```python
from build123d import *

# Parameters (mm, degrees)
BOSS_EXTRUDE1_DEPTH = 90
SKETCH3_R           = 13.36858006
BOSS_EXTRUDE2_DEPTH = 550
SKETCH4_R           = 30
CUT_EXTRUDE1_DEPTH  = 532.76


with BuildPart() as part:
    # Sketch2 → Boss-Extrude1 (new body)
    with BuildSketch(Plane(origin=(0, 0, 0), x_dir=(1, 0, 0), z_dir=(0, 1, 0))):
        with BuildLine():
            Line((-0.832718515, -13.342620159), (-2.264973014, -17.077408915))
            Line((-2.264973014, -17.077408915), (-9.734550526, -14.212899917))
            Line((-9.734550526, -14.212899917), (-8.302296027, -10.478111162))
            ThreePointArc((-8.302296027, -10.478111162), (4.786802233, 12.482205623), (-0.832718515, -13.342620159))
        make_face()
    extrude(amount=BOSS_EXTRUDE1_DEPTH)

    # Sketch3 → Boss-Extrude2 (add)
    with BuildSketch(Plane(origin=(0, 90, 0), x_dir=(1, 0, 0), z_dir=(0, 1, 0))):
        with Locations(Location((0, 0, 0), (0, 0, 231.608573475))):
            Circle(SKETCH3_R)
    extrude(amount=BOSS_EXTRUDE2_DEPTH)

    # Sketch4 → Cut-Extrude1 (cut)
    with BuildSketch(Plane(origin=(0, 640, 0), x_dir=(1, 0, 0), z_dir=(0, 1, 0))):
        Circle(SKETCH4_R)
    extrude(amount=-CUT_EXTRUDE1_DEPTH, mode=Mode.SUBTRACT)


solid = part.part
```
The listing builds one solid part. Answer for the finished solid, in the listing's coordinates (mm). A direction names the side the tool comes from. Give positions to 0.01 mm unless a question says otherwise; leave off trailing zeros. Loops run counter-clockwise (first coordinate to the right, second up) from the corner with the lowest first, then second, coordinate; pieces in that order, holes last. Notation, with made-up numbers: (49.25, -25.75) - (66.25, -25.75) arc R13 ccw to (66.25, -13.75) - close; hole circle Ø6 at (13.25, -30.5). An arc over 180 degrees is marked (long way). Return JSON: item names as keys, results as strings. Group by question number.
1. Straight lines are drawn through the part: line 1 (Z direction, x = 0.5, y = 11.5); line 2 (X direction, y = 30, z = 8.5); line 3 (Z direction, x = -5.75, y = 58). For each, find the intervals that lie inside material, in ascending order. Write a range as [from, to].
2. Which of the six approach directions +Z, -Z, +X, -X, +Y, -Y give full straight-line access (tool end or side, diameter ignored) to faces 4 (the flat face through (-5, 90, 14)), 5 (the flat face through (0, 0, 2))?
3. Given pin 1 Ø1 at (x, y) = (-6, 15.5) entering from -Z; pin 2 Ø12 at (y, z) = (22.5, 11) entering from +X; pin 3 Ø3 at (x, y) = (10.5, 47) entering from +Z, each flat-ended and moving along its own axis, determine where each tip first touches the part or whether it passes through.
4. Find section C-C (x = 8). Write down the section's boundary in (y, z).
5. Find section A-A (y = 10). Write down the section's boundary in (x, z).
6. Find section D-D (y = 95). Write down the section's boundary in (x, z), then the cut area to 3 significant figures.
7. Determine the mould class of faces 1 (the flat face through (-9.028, 44.37, 12.372)), 2 (the flat face through (-5.947, 44.37, 15.665)), 3 (the flat face through (0, 107.24, 0)) for opening direction Z: pulls with the +Z half, pulls with the -Z half, needs draft (parallel to the pull), parting line crosses it, or undercut.
8. Find section B-B (z = 11.5). Write down the section's boundary in (x, y).
Verdict:
{
 "1": {"line 1": "z = [-13.36, 13.36]", "line 2": "x = [-10.32, 10.32]", "line 3": "z = [-12.07, 15.74]"},
 "2": {"face 4": "+Z, -X, +Y", "face 5": "+Z, -Z, +X, -X, -Y"},
 "3": {"pin 1": "stops at z = -12.18", "pin 2": "stops at x = 12.4", "pin 3": "stops at z = 9.89"},
 "4": {"outline": "(0, -10.71) - (107.24, -10.71) - (107.24, 10.71) - (0, 10.71) - close"},
 "5": {"outline": "(-9.73, 14.21) - (-8.3, 10.48) arc R13.37 ccw (long way) to (-0.83, 13.34) - (-2.26, 17.08) - close"},
 "6": {"outline": "circle Ø26.74 at (0, 0)", "area": "561 mm^2"},
 "7": {"face 1": "undercut", "face 2": "pulls with the +Z half", "face 3": "needs draft"},
 "8": {"outline": "(-8.69, 0) - (6.82, 0) - (6.82, 107.24) - (-6.82, 107.24) - (-6.82, 90) - (-8.69, 90) - close"}
}
